from build123d import *

# Parameters (mm, degrees)
SKETCH1_R                       = 2.06
SKETCH1_W                       = 25
SKETCH1_H                       = 60
BOSS_EXTRUDE1_DEPTH             = 10
CUT_EXTRUDE1_START              = -6
SKETCH2_R                       = 3.06
SKETCH2_W                       = 27
SKETCH2_H                       = 62
CUT_EXTRUDE1_DEPTH              = 4
SKETCH3_R                       = 2
CUT_EXTRUDE2_DEPTH              = 7.5
CBORE_FOR_M8_SHCS1_D            = 9
CBORE_FOR_M8_SHCS1_CBORE_D      = 15
CBORE_FOR_M8_SHCS1_CBORE_DEPTH  = 8
F_6_0MM_CLEARANCE_DOWEL_HOLE1_D = 6


with BuildPart() as part:
    # Sketch1 → Boss-Extrude1 (new body)
    with BuildSketch(Plane.XY):
        with BuildLine():
            Line((22, 52), (22, -52))
            ThreePointArc((22, -52), (22.585786438, -53.414213562), (24, -54))
            Line((24, -54), (36, -54))
            Line((36, -54), (92.5, -54))
            ThreePointArc((92.5, -54), (93.914213562, -53.414213562), (94.5, -52))
            Line((94.5, -52), (94.5, 52))
            ThreePointArc((94.5, 52), (93.914213562, 53.414213562), (92.5, 54))
            Line((92.5, 54), (24, 54))
            ThreePointArc((24, 54), (22.585786438, 53.414213562), (22, 52))
        make_face()
        with Locations((29, -24)):
            Circle(SKETCH1_R, mode=Mode.SUBTRACT)
        with Locations((29, -9)):
            Circle(SKETCH1_R, mode=Mode.SUBTRACT)
        with Locations((58, 0)):
            Rectangle(SKETCH1_W, SKETCH1_H, mode=Mode.SUBTRACT)
    extrude(amount=-BOSS_EXTRUDE1_DEPTH)

    # Sketch2 → Cut-Extrude1 (cut)
    with BuildSketch(Plane.XY.offset(CUT_EXTRUDE1_START)):
        with Locations((29, -9)):
            Circle(SKETCH2_R)
        with Locations((29, -24)):
            Circle(SKETCH2_R)
        with Locations((58, 0)):
            Rectangle(SKETCH2_W, SKETCH2_H)
    extrude(amount=-CUT_EXTRUDE1_DEPTH, mode=Mode.SUBTRACT)

    # Sketch3 → Cut-Extrude2 (cut)
    with BuildSketch(Plane.XY):
        with Locations((27, 8.5)):
            Circle(SKETCH3_R)
        with Locations((27, 18.5)):
            Circle(SKETCH3_R)
        with Locations((74.5, 23)):
            Circle(SKETCH3_R)
        with Locations((74.5, -27)):
            Circle(SKETCH3_R)
    extrude(amount=-CUT_EXTRUDE2_DEPTH, mode=Mode.SUBTRACT)

    # CBORE for M8 SHCS1 (through all)
    with Locations(Plane(origin=(0, 0, 0), x_dir=(0.9063077870366375, -0.4226182617407263, 0), z_dir=(0, 0, 1))):
        with Locations((57.020425437, 72.930933649), (13.064497766, 52.433947955), (48.564431752, -23.695906156), (92.520359424, -3.198920462)):
            CounterBoreHole(CBORE_FOR_M8_SHCS1_D / 2, CBORE_FOR_M8_SHCS1_CBORE_D / 2, CBORE_FOR_M8_SHCS1_CBORE_DEPTH)

    # Ø6.0mm Clearance Dowel Hole1 (through all)
    with Locations(Plane(origin=(0, 0, 0), x_dir=(0.9063077870366375, -0.4226182617407263, 0), z_dir=(0, 0, 1))):
        with Locations((44.876877208, 70.578437869), (60.707979982, -21.343410377)):
            Hole(F_6_0MM_CLEARANCE_DOWEL_HOLE1_D / 2)


solid = part.part
Geometry: final body of the model. Coordinates: model frame, mm. A direction names the side the tool comes from. Round coordinates to 2 decimals unless told otherwise and drop trailing zeros. Loops run counter-clockwise (first coordinate to the right, second up) from the corner with the lowest first, then second, coordinate; pieces in that order, holes last. Notation, with made-up numbers: (16, 1.25) -> (63, 1.25) arc R18 cw to (63, 23.25) -> close; hole circle Ø1 at (50.25, 2). An arc over 180 degrees is marked (long way). One line per question, with ' | ' between items. Start each with the question number.
1. Section D-D on x = 37. Output: boundary loops of the cut face in (y, z).
2. Section A-A on y = 3.5. Output: boundary loops of the cut face in (x, z).
3. Mould query, pull axis X, two halves, no side actions, for faces 6 (the face through (22.57, -53.4, -4.93)), 7 (the face through (42, 1, 0)), 8 (the face through (45.5, 0, -3)). Classes: pulls with the +X half, pulls with the -X half, needs draft (parallel to the pull), parting line crosses it, or undercut.
4. Section C-C on y = -9. Output: boundary loops of the cut face in (x, z).
5. Section B-B on x = 51.5. Output: boundary loops of the cut face in (y, z).
6. Contact query for flat-ended pins moving along their axis: pin 1 (16.5 mm diameter, centred on x = 35.5, y = -39.5, fed in from +Z); pin 2 (7.5 mm diameter, centred on x = 81.5, y = -38.5, fed in from +Z). Output: stop coordinate, or through.
7. Set-up query: faces 1 (the face through (93.9, -53.43, -4.93)), 2 (the face through (87, -44, -8)), 3 (the face through (22.6, 53.43, -4.93)), 4 (the face through (58, 30, -3)), 5 (the face through (26.745, -21.932, -7.972)). Return all of +Z, -Z, +X, -X, +Y, -Y with unobstructed straight access to the full face (end or side cutting, diameter ignored); none if empty.
8. Line query: line 1 along Y through (x, z) = (83, -2.5); line 2 along Y through (x, z) = (82.5, -9.5); line 3 along X through (y, z) = (29, -2). Output: solid intervals per line, ascending. Write a range as [from, to].
Returned:
1) outline: (-54, -10) -> (-45.35, -10) -> (-45.35, -8) -> (-48.87, -8) -> (-48.87, 0) -> (-54, 0) -> close; (-38.65, -10) -> (38.65, -10) -> (38.65, -8) -> (35.13, -8) -> (35.13, 0) -> (-35.13, 0) -> (-35.13, -8) -> (-38.65, -8) -> close; (45.35, -10) -> (54, -10) -> (54, 0) -> (48.87, 0) -> (48.87, -8) -> (45.35, -8) -> close
2) outline: (22, -10) -> (44.5, -10) -> (44.5, -6) -> (45.5, -6) -> (45.5, 0) -> (22, 0) -> close; (70.5, -6) -> (71.5, -6) -> (71.5, -10) -> (94.5, -10) -> (94.5, 0) -> (70.5, 0) -> close
3) face 6: pulls with the -X half | face 7: needs draft | face 8: undercut
4) outline: (22, -10) -> (25.94, -10) -> (25.94, -6) -> (26.94, -6) -> (26.94, 0) -> (22, 0) -> close; (31.06, -6) -> (32.06, -6) -> (32.06, -10) -> (44.5, -10) -> (44.5, -6) -> (45.5, -6) -> (45.5, 0) -> (31.06, 0) -> close; (70.5, -6) -> (71.5, -6) -> (71.5, -10) -> (94.5, -10) -> (94.5, 0) -> (70.5, 0) -> close
5) outline: (-54, -10) -> (-31, -10) -> (-31, -6) -> (-30, -6) -> (-30, 0) -> (-54, 0) -> close; (30, -6) -> (31, -6) -> (31, -10) -> (54, -10) -> (54, 0) -> (30, 0) -> close
6) pin 1: stops at z = 0 | pin 2: stops at z = -8
7) face 1: +Z, -Z, +X, -Y | face 2: +Z | face 3: +Z, -Z, -X, +Y | face 4: +Z, -Z | face 5: -Z
8) line 1: y = [-54, -49.48], [-34.52, 34.52], [49.48, 54] | line 2: y = [-54, -46.5], [-37.5, 37.5], [46.5, 54] | line 3: x = [22, 45.5], [70.5, 94.5]
